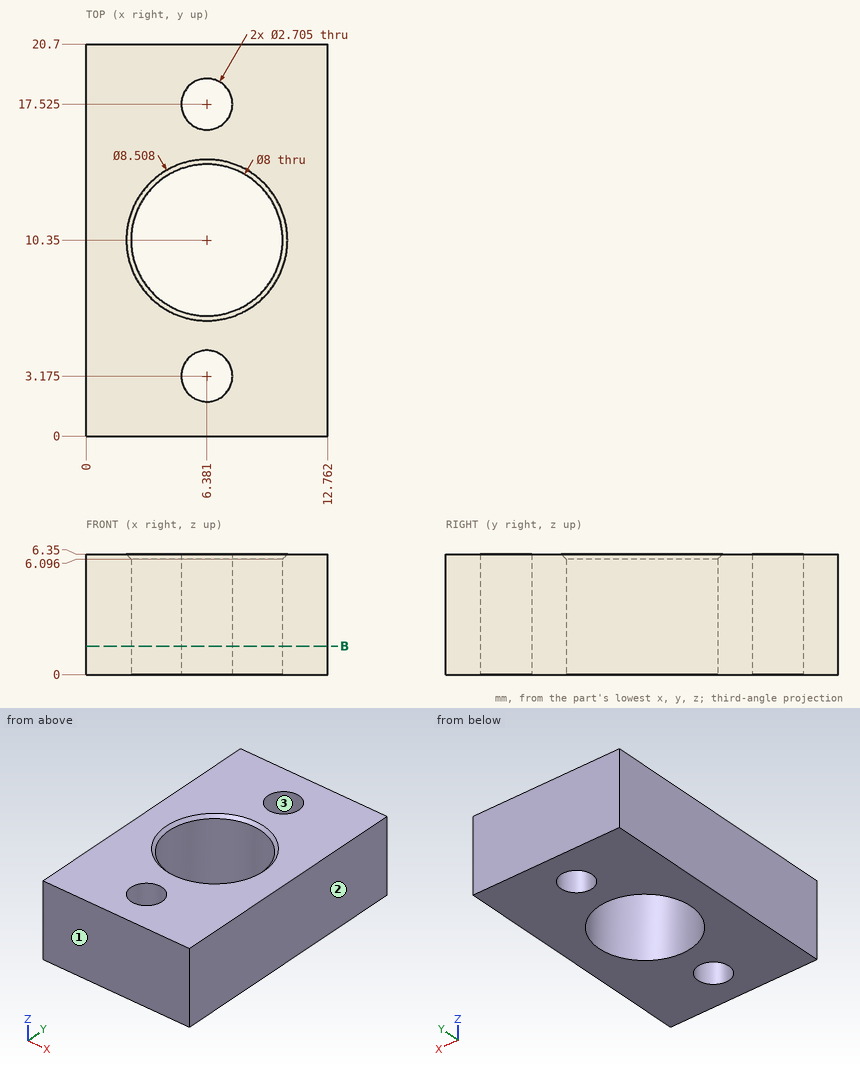
For this review, use the dimensioned drawing (mm, ordinates from the lowest corner) and the shaded views. Round coordinates to 2 decimals unless told otherwise and drop trailing zeros. Use a Markdown table: item, result. Add a question column.
Item 1: Add section B-B, the plane z = 1.5. State how many separate pieces and enclosed holes the cut face has.
Item 2: Mouldability with a two-part tool opening along Y and no side actions: class the marked faces 1, 2 and 3 as released by +Y, released by -Y, zero draft, split by the parting line, or undercut.
Item 3: Insertion check: pin 1 (4 mm diameter, centred on x = 8, y = 10.5, fed in from -Z). The pin has a flat end and moves straight along its axis. Give the tip position at first contact, or say it passes through.
Item 4: To check wall thickness, follow line 1 along Y through (x, z) = (6, 1.75); line 2 along X through (y, z) = (3.25, 1.5); line 3 along Y through (x, z) = (4.5, 3.25). State the ranges of each line that lie inside material, in increasing order.
Geometry results:
| question | item | result |
|---|---|---|
| 1 | separate pieces | 1 |
| 1 | enclosed holes | 3 |
| 2 | face 1 | released by -Y |
| 2 | face 2 | zero draft |
| 2 | face 3 | undercut |
| 3 | pin 1 | passes through |
| 4 | line 1 | y = 0 to 1.88, 4.47 to 6.37, 14.33 to 16.23, 18.82 to 20.7 |
| 4 | line 2 | x = 0 to 5.03, 7.73 to 12.76 |
| 4 | line 3 | y = 0 to 6.82, 13.88 to 20.7 |
